Build history of the part. All positions in model axes, mm. Face numbers are marked on the shaded views. A direction names the side the tool comes from. Give positions to 0.01 mm unless a question says otherwise; leave off trailing zeros. Order: outer loops, then holes, each group sorted by start corner. A loop starts at its lowest first (then second) coordinate and runs counter-clockwise, first axis right, second up. Notation, with made-up numbers: M 23.25,-13.5 L 47.25,-13.5 A19 cw 47.25,-2.5 Z; hole C 52,16.5 d9. An arc over 180 degrees is marked long. One line per item, written item: value.
from build123d import *

# Parameters (mm, degrees)
SKETCH1_R           = 5
SKETCH1_R_2         = 1.75
BOSS_EXTRUDE1_DEPTH = 4
SKETCH2_W           = 4
SKETCH2_H           = 10
BOSS_EXTRUDE2_DEPTH = 27
SKETCH3_R           = 1.75
CUT_EXTRUDE1_DEPTH  = 4
FILLET1_R           = 2
FILLET2_R           = 2


with BuildPart() as part:
    # Sketch1 → Boss-Extrude1 (new body)
    # profile 1 of 3: a face of its own
    with BuildSketch(Plane(origin=(0, 0, 0), x_dir=(1, 0, 0), z_dir=(0, 1, 0))):
        with Locations((-8, 0)):
            Circle(SKETCH1_R)
        with Locations(Location((-8, 0, 0), (0, 0, 270))):
            Circle(SKETCH1_R_2, mode=Mode.SUBTRACT)
    # profile 2 of 3: a face of its own
    with BuildSketch(Plane(origin=(0, 0, 0), x_dir=(1, 0, 0), z_dir=(0, 1, 0))):
        with BuildLine():
            Line((8, 5), (-8, 5))
            ThreePointArc((-8, 5), (-4.464466094, 3.535533906), (-3, 0))
            ThreePointArc((-3, 0), (-4.464466094, -3.535533906), (-8, -5))
            Line((-8, -5), (8, -5))
            ThreePointArc((8, -5), (3, 0), (8, 5))
        make_face()
    # profile 3 of 3: a face of its own
    with BuildSketch(Plane(origin=(0, 0, 0), x_dir=(1, 0, 0), z_dir=(0, 1, 0))):
        with Locations((8, 0)):
            Circle(SKETCH1_R)
        with Locations(Location((8, 0, 0), (0, 0, 270))):
            Circle(SKETCH1_R_2, mode=Mode.SUBTRACT)
    extrude(amount=BOSS_EXTRUDE1_DEPTH)

    # Sketch2 → Boss-Extrude2 (add)
    with BuildSketch(Plane(origin=(0, 4, 0), x_dir=(1, 0, 0), z_dir=(0, 1, 0))):
        Rectangle(SKETCH2_W, SKETCH2_H)
    extrude(amount=BOSS_EXTRUDE2_DEPTH)

    # Sketch3 → Cut-Extrude1 (cut)
    with BuildSketch(Plane(origin=(2, 0, 0), x_dir=(0, 0, -1), z_dir=(1, 0, 0))):
        with BuildLine():
            Line((-5, 31), (-5, 26))
            ThreePointArc((-5, 26), (-3.535533906, 29.535533906), (0, 31))
            Line((0, 31), (-5, 31))
        make_face()
        with BuildLine():
            ThreePointArc((0, 31), (3.535533906, 29.535533906), (5, 26))
            Line((5, 26), (5, 31))
            Line((5, 31), (0, 31))
        make_face()
        with Locations((0, 26)):
            Circle(SKETCH3_R)
    extrude(amount=-CUT_EXTRUDE1_DEPTH, mode=Mode.SUBTRACT)

    # Fillet1
    fillet1_edges = [part.edges().sort_by_distance(p)[0] for p in [
        (2, 4, 0),
    ]]
    fillet(fillet1_edges, radius=FILLET1_R)

    # Fillet2
    fillet2_edges = [part.edges().sort_by_distance(p)[0] for p in [
        (-2, 4, 0),
    ]]
    fillet(fillet2_edges, radius=FILLET2_R)


solid = part.part
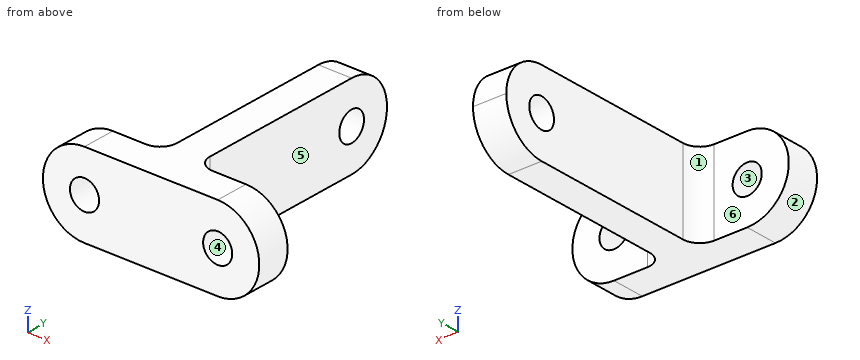
1) Drill centre lines: probe 1 along X at (y, z) = (1.3, 0); probe 2 along X at (y, z) = (14, -1.25); probe 3 along Y at (x, z) = (6.25, -4.5). Where is each one in solid material? Low to high. Write a range as from..to.
Check values:
probe 1: -13..-9.75, -6.25..6.25, 9.75..13
probe 2: -2..2
probe 3: 0..4
2) Tool access for the marked faces 4, 5 and 6: list every direction of +Z, -Z, +X, -X, +Y, -Y with a clear straight run to the whole face (end or side of a thin tool).
Check values:
face 4: +Y, -Y
face 5: +Z, -Z, +X, +Y
face 6: +Z, -Z, -X, +Y
3) Saw through at A-A, the plane x = 0. Write the cut outline in (y, z), then the cut area to 3 significant figures.
Check values:
outline: M 0,-5 L 26,-5 A5 ccw 26,5 L 0,5 Z; hole C 26,0 d3.5
area: 290 mm^2
4) Saw through at C-C, the plane x = 9.25. Write the cut outline in (y, z).
Check values:
outline: M 0,-4.84 L 4,-4.84 L 4,-1.22 L 0,-1.22 Z; M 0,1.22 L 4,1.22 L 4,4.84 L 0,4.84 Z
5) Pin check, flat tips, straight feed: pin 1 (3 mm diameter, centred on y = 27.5, z = 3.5, fed in from +X); pin 2 (8 mm diameter, centred on x = 5, y = 5, fed in from +Z); pin 3 (3 mm diameter, centred on x = -4.5, y = 21, fed in from -Z); pin 4 (4.5 mm diameter, centred on x = 8.5, z = 0, fed in from +Y). Stop position of each tip, or through.
Check values:
pin 1: x = 2
pin 2: z = 5
pin 3: through
pin 4: y = 4
6) Saw through at D-D, the plane y = 18.5. Write the cut outline in (x, z).
Check values:
outline: M -2,-5 L 2,-5 L 2,5 L -2,5 Z
7) Mould opens along Z. For the marked faces 1, 2 and 3 say: released by +Z, released by -Z, zero draft, split by the parting line, or undercut.
Check values:
face 1: zero draft
face 2: split by the parting line
face 3: undercut
8) Saw through at B-B, the plane z = 4. Write the cut outline in (x, y), then the cut area to 3 significant figures.
Check values:
outline: M -11,0 L 11,0 L 11,4 L 4,4 A2 cw 2,6 L 2,29 L -2,29 L -2,6 A2 cw -4,4 L -11,4 Z
area: 190 mm^2
